from build123d import *

# Parameters (mm, degrees)
SKETCH1_R           = 1.5
BOSS_EXTRUDE1_DEPTH = 2


with BuildPart() as part:
    # Sketch1 → Boss-Extrude1 (new body)
    with BuildSketch(Plane(origin=(0, 0, 0), x_dir=(1, 0, 0), z_dir=(0, 1, 0))):
        with BuildLine():
            Line((60, 15.491933385), (60, 8))
            ThreePointArc((60, 8), (58.828427125, 5.171572875), (56, 4))
            Line((56, 4), (-59, 4))
            ThreePointArc((-59, 4), (-59.707106781, 3.707106781), (-60, 3))
            Line((-60, 3), (-60, -3))
            ThreePointArc((-60, -3), (-59.707106781, -3.707106781), (-59, -4))
            Line((-59, -4), (56, -4))
            ThreePointArc((56, -4), (58.828427125, -5.171572875), (60, -8))
            Line((60, -8), (60, -15.491933385))
            ThreePointArc((60, -15.491933385), (61.550510257, -18.654211045), (65, -19.364916731))
            ThreePointArc((65, -19.364916731), (80, 0), (65, 19.364916731))
            ThreePointArc((65, 19.364916731), (61.550510257, 18.654211045), (60, 15.491933385))
        make_face()
        with Locations(Location((-55, 0, 0), (0, 0, 270))):
            Circle(SKETCH1_R, mode=Mode.SUBTRACT)
    extrude(amount=BOSS_EXTRUDE1_DEPTH)


solid = part.part
Design review of the part built by this model. Coordinates are the model's own, in mm. Give positions to 0.01 mm unless a question says otherwise; leave off trailing zeros. Loops run counter-clockwise (first coordinate to the right, second up) from the corner with the lowest first, then second, coordinate; pieces in that order, holes last. Notation, with made-up numbers: M 20,20.25 L 44,20.25 A18 ccw 44,38.25 Z; hole C 28.5,-27 d3. An arc over 180 degrees is marked long. Write item = value, one per line.
Q1. We need section C-C (z = 0). Give the boundary of the cut face in (x, y).
Output values:
outline = M -60,0 L -56.5,0 L -56.5,2 L -60,2 Z; M -53.5,0 L 80,0 L 80,2 L -53.5,2 Z
Q2. To check wall thickness, follow line 1 (X direction, y = 0.4, z = 0); line 2 (Z direction, x = 56, y = 1.05); line 3 (X direction, y = 0.75, z = 1). State the ranges of each line that lie inside material, in increasing order. Write a range as [from, to].
Output values:
line_1 = [-60, -56.5], [-53.5, 80]
line_2 = [-4, 4]
line_3 = [-60, -56.12], [-53.88, 79.97]
Q3. We need section B-B (y = 1.2). Give the boundary of the cut face in (x, z), plus the area to 3 significant figures.
Output values:
outline = M -60,-3 A1 ccw -59,-4 L 56,-4 A4 cw 60,-8 L 60,-15.49 A4 ccw 65,-19.36 A20 ccw 65,19.36 A4 ccw 60,15.49 L 60,8 A4 cw 56,4 L -59,4 A1 ccw -60,3 Z; hole C -55,0 d3
area = 1,580 mm^2
Q4. We need section D-D (x = 28). Give the boundary of the cut face in (y, z), plus the area to 3 significant figures.
Output values:
outline = M 0,-4 L 2,-4 L 2,4 L 0,4 Z
area = 16.0 mm^2
Q5. Draft analysis for pull direction Z (two halves, no side actions). For faces 1 (the cylindrical face through (61.51, 0.99, 18.62)), 2 (the cylindrical face through (58.859, 0.986, -5.203)), 3 (the cylindrical face through (-53.99, 0.99, -1.11)), state which applies: +Z half, -Z half, draft (parallel to the pull), parting line (faces both ways), or undercut.
Output values:
face_1 = +Z half
face_2 = -Z half
face_3 = undercut
Q6. We need section A-A (x = -55). Give the boundary of the cut face in (y, z), plus the area to 3 significant figures.
Output values:
outline = M 0,-4 L 2,-4 L 2,-1.5 L 0,-1.5 Z; M 0,1.5 L 2,1.5 L 2,4 L 0,4 Z
area = 10.0 mm^2
Q7. Insertion check: pin 1 (0.6 mm diameter, centred on y = 0.5, z = 13, fed in from -X); pin 2 (1 mm diameter, centred on x = 15.5, y = 0.5, fed in from +Z); pin 3 (4 mm diameter, centred on x = -55, z = 0, fed in from +Y); pin 4 (1 mm diameter, centred on y = 1.5, z = 10, fed in from +X). Each pin has a flat end and moves straight along its axis. Give the tip position at first contact, or say it passes through.
Output values:
pin_1 = 60
pin_2 = 4
pin_3 = 2
pin_4 = 77.6
